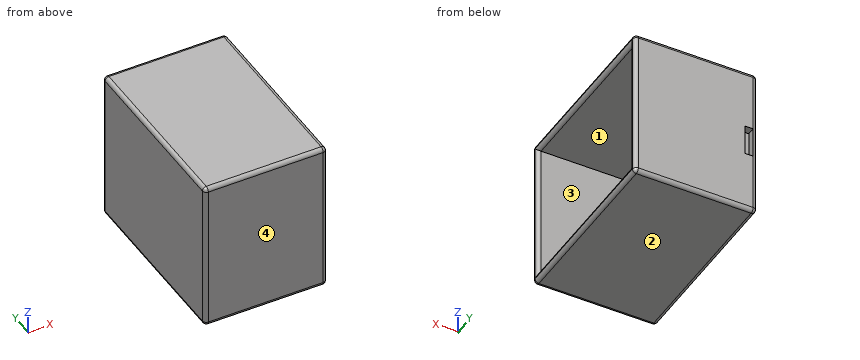
Autodesk Inventor part; units mm, degrees
ref_plane "YZ Plane" through (0, 0, 0) normal (1, 0, 0) x (0, 1, 0)
ref_plane "XZ Plane" through (0, 0, 0) normal (0, 1, 0) x (-1, 0, 0)
ref_plane "XY Plane" through (0, 0, 0) normal (0, 0, 1) x (1, 0, 0)
sketch "Sketch1" plane through (0, 0, 0) normal (0, 0, 1) x (1, 0, 0)
  line L0 (0, 0) -> (101.6, 0)
  line L1 (101.6, 0) -> (101.6, 152.4)
  line L2 (101.6, 152.4) -> (0, 152.4)
  line L3 (0, 152.4) -> (0, 0)
  dimension "d0" = 101.6
  dimension "d1" = 152.4
sketch "Sketch2" plane through (0, 0, 0) normal (0, 0, 1) x (1, 0, 0)
  point P0 (0, 0)
sketch "Sketch3" plane through (0, 0, 0) normal (0, 0, 1) x (1, 0, 0)
  point P0 (0, 0)
extrude "Extrusion1" add sketch "Sketch1" along normal blind 127
sketch "Sketch4" plane through (101.6, 0, 0) normal (1, 0, 0) x (0, 0, -1)
  line L0 (0, 0) -> (-127, 0)
  line L1 (0, 0) -> (-6.35, 0)
  line L2 (-6.35, 0) -> (-6.35, 6.35)
  line L3 (-6.35, 6.35) -> (0, 6.35)
  line L4 (0, 6.35) -> (0, 0)
  line L5 (-6.35, 6.35) -> (-120.65, 6.35)
  line L6 (-120.65, 6.35) -> (-120.65, 146.05)
  line L7 (-120.65, 146.05) -> (-6.35, 146.05)
  line L8 (-6.35, 146.05) -> (-6.35, 6.35)
  dimension "d4" = 6.35
  dimension "d5" = 6.35
  dimension "d6" = 114.3
  dimension "d7" = 139.7
extrude "Extrusion2" cut sketch "Sketch4" against normal blind 95.25 contours L5 L6 L7 L8
fillet "Fillet1" radius 3.175 8 edges at (101.6, 146.05, 63.5) (101.6, 152.4, 63.5) (101.6, 76.2, 127) (101.6, 76.2, 120.65) (101.6, 76.2, 6.35) (101.6, 76.2, 0) (101.6, 6.35, 63.5) (101.6, 0, 63.5)
fillet "Fillet2" radius 3.175 8 edges at (100.6701, 151.4701, 126.0701) (49.2126, 152.4, 127) (100.6701, 151.4701, 0.9299) (49.2126, 152.4, 0) (100.6701, 0.9299, 126.0701) (49.2126, 0, 127) (100.6701, 0.9299, 0.9299) (49.2126, 0, 0)
fillet "Fillet3" radius 3.175 8 edges at (0, 0.9299, 0.9299) (0, 0, 63.5) (0, 0.9299, 126.0701) (0, 76.2, 127) (0, 151.4701, 126.0701) (0, 152.4, 63.5) (0, 151.4701, 0.9299) (0, 76.2, 0)
sketch "Sketch5" plane through (6.35, 6.35, 6.35) normal (0, 0, 1) x (1, 0, 0)
  line L0 (92.075, 0) -> (0, 0)
  arc A0 (95.25, -3.175) -> (92.075, 0) centre (92.075, -3.175) ccw
  line L1 (92.075, 0) -> (89.535, 0)
  line L2 (92.075, 0) -> (94.615, 0) construction
  line L3 (91.2996, 0) -> (88.936, -0.9299)
  point P0 (-6.35, -6.35)
sketch "Sketch6" plane through (6.35, 6.35, 6.35) normal (0, 0, 1) x (1, 0, 0)
  point P0 (-6.35, -6.35)
sketch "Sketch7" plane through (98.425, 152.4, 123.825) normal (0, 1, 0) x (1, 0, 0)
  line L0 (-95.25, 120.65) -> (0, 120.65)
  line L1 (-95.25, 120.65) -> (-95.25, 73.025)
  line L2 (0, 0) -> (-95.25, 0)
  arc A0 (-98.425, 0) -> (-95.25, -3.175) centre (-95.25, 0) ccw
  line L3 (-92.075, 3.175) -> (-92.075, 117.475)
  line L4 (-95.25, 0) -> (-98.425, 0)
  line L5 (-95.25, 0) -> (-95.25, 47.625)
  line L6 (-95.25, 0) -> (-95.25, 120.65)
  line L7 (-95.25, 73.025) -> (-95.25, 47.625)
  line L8 (-95.25, 47.625) -> (-91.44, 47.625)
  line L9 (-91.44, 47.625) -> (-91.44, 73.025)
  line L10 (-91.44, 73.025) -> (-95.25, 73.025)
  point P0 (-98.425, 123.825)
  point P1 (-92.075, 73.025)
  point P2 (-92.075, 47.625)
  dimension "d17" = 47.625
  dimension "d20" = 47.625
  dimension "d21" = 3.81
sketch "Sketch8" plane through (98.425, 152.4, 123.825) normal (0, 1, 0) x (1, 0, 0)
  point P0 (-98.425, 123.825)
extrude "Extrusion3" cut sketch "Sketch7" against normal blind 6.604 contours L8 L6 L10 L3
sketch "Sketch9" plane through (98.425, 152.4, 123.825) normal (0, 1, 0) x (1, 0, 0)
  line L0 (-95.25, 73.025) -> (-92.075, 73.025)
  line L1 (-92.075, 73.025) -> (-92.075, 47.625)
  line L2 (-92.075, 73.025) -> (-92.075, 47.625)
  line L3 (-92.075, 47.625) -> (-88.265, 47.625)
  line L4 (-88.265, 47.625) -> (-88.265, 73.025)
  line L5 (-88.265, 73.025) -> (-92.075, 73.025)
  point P0 (-98.425, 123.825)
  dimension "d24" = 3.81
extrude "Extrusion4" cut sketch "Sketch9" against normal blind 7.62
properties part number "box"
Part model, mm, in its own coordinate system. Face numbers are marked on the shaded views. Give positions to 0.01 mm unless a question says otherwise; leave off trailing zeros. Order: outer loops, then holes, each group sorted by start corner. A loop starts at its lowest first (then second) coordinate and runs counter-clockwise, first axis right, second up. Notation, with made-up numbers: (69.25, 33.25) - (125.25, 33.25) arc R20 ccw to (125.25, 58.25) - close; hole circle Ø7 at (42, 34.5). An arc over 180 degrees is marked (long way). Use one line per item in the form item = value.
Item 1: Two-plate mould, pull along Z, no slides. Class the marked faces 1, 2, 3 and 4: released by +Z, released by -Z, zero draft, split by the parting line, or undercut.
Solution:
face_1 = undercut
face_2 = released by -Z
face_3 = undercut
face_4 = zero draft
Item 2: Slice it at B-B on x = 56. Give the cut face in (y, z) (3 decimals), and give its area (3 significant figures).
Solution:
outline = (0, 3.175) arc R3.175 ccw to (3.175, 0) - (149.225, 0) arc R3.175 ccw to (152.4, 3.175) - (152.4, 123.825) arc R3.175 ccw to (149.225, 127) - (3.175, 127) arc R3.175 ccw to (0, 123.825) - close; hole (6.35, 6.35) - (146.05, 6.35) - (146.05, 120.65) - (6.35, 120.65) - close
area = 3,380 mm2
Item 3: Pin check, flat tips, straight feed: pin 1 Ø2 at (y, z) = (54, 20.5) entering from +X; pin 2 Ø3.5 at (x, z) = (5.5, 60) entering from +Y. Stop position of each tip, or through.
Solution:
pin_1 = 6.35
pin_2 = 145.8
Item 4: Probe probe 1 along Z at (x, y) = (40, 43.5); probe 2 along Y at (x, z) = (70.5, 108); probe 3 along X at (y, z) = (45.5, 55). List the from-to ranges inside material, lowest first. Write a range as from..to.
Solution:
probe_1 = 0..6.35, 120.65..127
probe_2 = 0..6.35, 146.05..152.4
probe_3 = 0..6.35
